from build123d import *

# Parameters (mm, degrees)
F0_R     = 6.35
F1_DEPTH = 9.525
F2_D     = 7.9375


with BuildPart() as f1:
    # F0 (on Front) → F1 (new body)
    with BuildSketch(Plane.XZ):
        with BuildLine():
            Line((76.2, -28.1686), (76.2, 28.1686))
            ThreePointArc((76.2, 28.1686), (75.6890722442, 30.6641430927), (74.2385085583, 32.7580980808))
            Line((74.2385085583, 32.7580980808), (-49.0417475627, 150.6394980808))
            ThreePointArc((-49.0417475627, 150.6394980808), (-51.0660239849, 151.9434630233), (-53.4302561211, 152.4))
            Line((-53.4302561211, 152.4), (-69.8495712494, 152.4))
            ThreePointArc((-69.8495712494, 152.4), (-74.3398508885, 150.5399764769), (-76.1995712349, 146.0495712639))
            Line((-76.1995712349, 146.0495712639), (-76.197856327, 120.6501128256))
            ThreePointArc((-76.197856327, 120.6501128256), (-74.3380242773, 116.1600246552), (-69.8479691527, 114.3001128266))
            Line((-69.8479691527, 114.3001128266), (-50.7979691557, 114.2997743497))
            ThreePointArc((-50.7979691557, 114.2997743497), (-46.3078741417, 112.4398226308), (-44.4480819823, 107.9496615251))
            Line((-44.4480819823, 107.9496615251), (-44.4519180538, -107.9503384408))
            ThreePointArc((-44.4519180538, -107.9503384408), (-46.3118298823, -112.4403935654), (-50.8019180528, -114.3002256152))
            Line((-50.8019180528, -114.3002256152), (-69.850000004, -114.3002256152))
            ThreePointArc((-69.850000004, -114.3002256152), (-74.3400482968, -116.1600177883), (-76.2, -120.65))
            Line((-76.2, -120.65), (-76.2, -146.05))
            ThreePointArc((-76.2, -146.05), (-74.3401280605, -150.5401280605), (-69.85, -152.4))
            Line((-69.85, -152.4), (-48.3453483747, -152.4))
            ThreePointArc((-48.3453483747, -152.4), (-45.9191803183, -151.9182372619), (-43.861150015, -150.5460499408))
            Line((-43.861150015, -150.5460499408), (74.2293103448, -32.7668758621))
            ThreePointArc((74.2293103448, -32.7668758621), (75.6865709406, -30.669987546), (76.2, -28.1686))
        make_face()
        with Locations((-57.15, -133.3500654614)):
            Circle(F0_R, mode=Mode.SUBTRACT)
        with Locations((-57.1459382772, 133.333966136)):
            Circle(F0_R, mode=Mode.SUBTRACT)
        with BuildLine():
            ThreePointArc((42.4925458609, 23.8269667194), (40.1083667194, 30.1260541391), (46.4074541391, 32.5102332806))
            ThreePointArc((46.4074541391, 32.5102332806), (67.411691348, 0), (46.4074541391, -32.5102332806))
            ThreePointArc((46.4074541391, -32.5102332806), (40.1083667194, -30.1260541391), (42.4925458609, -23.8269667194))
            ThreePointArc((42.4925458609, -23.8269667194), (57.886691348, 0), (42.4925458609, 23.8269667194))
        make_face(mode=Mode.SUBTRACT)
    extrude(amount=F1_DEPTH)

    # F2 (through all)
    with Locations(Plane(origin=(0, 0, 0), x_dir=(1, 0, 0), z_dir=(0, 1, 0))):
        with Locations((31.75, 0), (-31.7444263581, -69.8504291124), (-31.75, 69.85)):
            Hole(F2_D / 2)


solid = f1.part
Could you check a few things on this model? Use its own coordinates, in mm. A direction names the side the tool comes from. Give positions to 0.01 mm unless a question says otherwise; leave off trailing zeros. Write each loop counter-clockwise with the first axis right and the second up, starting at its lowest first coordinate (ties: lowest second). Pieces come first, ordered by that corner, then holes. Notation, with made-up numbers: (63.5, 39.25) -> (106.5, 39.25) arc R16 ccw to (106.5, 59.25) -> close; hole circle Ø7 at (27, 77). An arc over 180 degrees is marked (long way). Write each question's results on one line, items separated by ' | '. Start each with the question number.
Q1. Suppose I cut it at D-D, the plane x = -31.75. List the corners of the cut face in (y, z) for me (3 decimals).
Q2. Suppose I cut it at A-A, the plane z = 0. List the corners of the cut face in (x, y) for me (3 decimals).
Q3. Suppose I cut it at B-B, the plane y = -1.5. State how many separate pieces and enclosed holes the cut face has, and give its area (3 significant figures).
Q4. I'm going to push flat-ended pins straight in: pin 1 Ø5 at (x, y) = (43.5, -8.5) entering from +Z; pin 2 Ø2 at (y, z) = (-1.5, -83) entering from -X; pin 3 Ø5 at (x, y) = (-27, -7) entering from +Z. Where does each tip first touch, or does it pass through?
Q5. We'd pull the mould along X, two halves only. Please class faces 1 (the face through (40.15, -4.7, -30.22)), 2 (the face through (14.36, -4.7, -92.48)), 3 (the face through (-74.29, -4.7, 150.59)): +X half, -X half, draft (parallel to the pull), parting line (faces both ways), or undercut.
Q6. Which directions (+Z, -Z, +X, -X, +Y, -Y) give clear straight access to the entire face, cutting with the end or side of a thin tool? Please do faces 4 (the face through (-74.39, -4.7, -150.49)), 5 (the face through (-60, -5, -114.3)), 6 (the face through (67.407, -4.696, 0.573)).
Q7. I need wall thicknesses on probe 1 along Z at (x, y) = (-57.15, -1.75); probe 2 along Z at (x, y) = (-31, -4.75); probe 3 along Z at (x, y) = (48.5, -4.5). Which ranges of each line are inside material? Lowest first, please.
Q8. Suppose I cut it at C-C, the plane x = 31.75. List the corners of the cut face in (y, z) for me (3 decimals).
Outcome:
1) outline: (-9.525, -138.467) -> (0, -138.467) -> (0, -73.819) -> (-9.525, -73.819) -> close; (-9.525, -65.881) -> (0, -65.881) -> (0, 65.882) -> (-9.525, 65.882) -> close; (-9.525, 73.819) -> (0, 73.819) -> (0, 134.105) -> (-9.525, 134.105) -> close
2) outline: (-44.45, -9.525) -> (27.781, -9.525) -> (27.781, 0) -> (-44.45, 0) -> close; (35.719, -9.525) -> (57.887, -9.525) -> (57.887, 0) -> (35.719, 0) -> close; (67.412, -9.525) -> (76.2, -9.525) -> (76.2, 0) -> (67.412, 0) -> close
3) separate pieces: 1 | enclosed holes: 6 | area: 22,900 mm2
4) pin 1: z = 64.54 | pin 2: x = -44.45 | pin 3: z = 131.95
5) face 1: undercut | face 2: +X half | face 3: -X half
6) face 4: -Z, -X, +Y, -Y | face 5: -X, +Y, -Y | face 6: +Y, -Y
7) probe 1: -152.4 to -139.7, -127 to -114.3, 114.3 to 126.98, 139.68 to 152.4 | probe 2: -137.72 to -73.75, -65.95 to 65.95, 73.75 to 133.39 | probe 3: -58.43 to -31.48, -20.06 to 20.06, 31.48 to 57.37
8) outline: (-9.525, -75.134) -> (0, -75.134) -> (0, -3.969) -> (-9.525, -3.969) -> close; (-9.525, 3.969) -> (0, 3.969) -> (0, 73.386) -> (-9.525, 73.386) -> close
